Here's how the part is built. I have some questions about the finished solid (model axes, mm). Face numbers are marked on the shaded views. Round coordinates to 2 decimals unless told otherwise and drop trailing zeros. Loops run counter-clockwise (first coordinate to the right, second up) from the corner with the lowest first, then second, coordinate; pieces in that order, holes last. Notation, with made-up numbers: (18, 19.5) -> (36, 19.5) arc R26 ccw to (36, 40.5) -> close; hole circle Ø3 at (57, 55). An arc over 180 degrees is marked (long way). Use one line per item in the form item = value. Start each with the question number.
Item 1: If we section it at D-D (z = 0.25): Write out the boundary of the cut face in (x, y), then the cut area to 3 significant figures.
Item 2: If we section it at A-A (y = 8): Write out the boundary of the cut face in (x, z), then the cut area to 3 significant figures.
Item 3: If we section it at B-B (z = 4.75): Write out the boundary of the cut face in (x, y).
Item 4: If we section it at C-C (x = 27.5): Write out the boundary of the cut face in (y, z), then the cut area to 3 significant figures.
Item 5: I'm going to push flat-ended pins straight in: pin 1 Ø6 at (x, z) = (18.5, -3) entering from -Y; pin 2 Ø8 at (x, y) = (8, 8) entering from +Z. Where does each tip first touch, or does it pass through?
Item 6: Thinking about a two-plate mould opening in Y: for the marked faces 1, 2 and 3, which applies, released by +Y, released by -Y, zero draft, split by the parting line, or undercut?
Item 7: If I drill on L1, parallel to X at y = 36, z = -4.5; L2, parallel to X at y = 8, z = 2.75; L3, parallel to Y at x = 45, z = -5, over which ranges is the centre line in solid material (lowest first)? Write a range as [from, to].
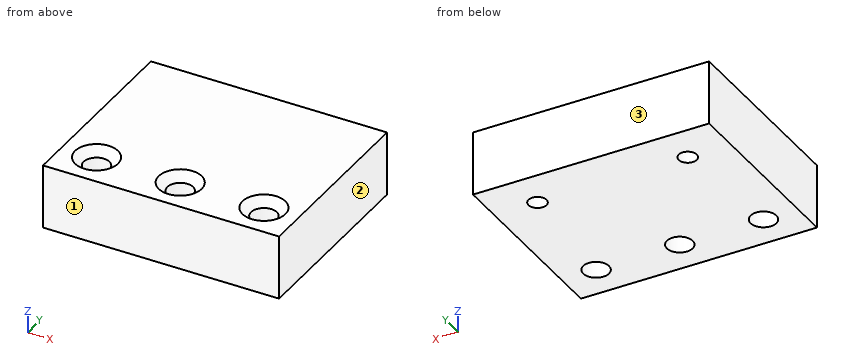
```python
from build123d import *

# Parameters (mm, degrees)
SKETCH1_W                       = 55
SKETCH1_H                       = 45
BOSS_EXTRUDE1_DEPTH             = 7.5
F_6_0MM_DOWEL_HOLE1_D           = 6
F_6_0MM_DOWEL_HOLE1_CSINK_D     = 10
F_6_0MM_DOWEL_HOLE1_CSINK_ANGLE = 90
TAP_DRILL_FOR_M5X0_8_TAP2_D     = 4.2
TAP_DRILL_FOR_M5X0_8_TAP2_DEPTH = 10
TAP_DRILL_FOR_M5X0_8_TAP2_TIP   = 1.2618073


with BuildPart() as part:
    # Sketch1 → Boss-Extrude1 (new body, symmetric)
    with BuildSketch(Plane.XY):
        with Locations((27.5, 22.5)):
            Rectangle(SKETCH1_W, SKETCH1_H)
    extrude(amount=BOSS_EXTRUDE1_DEPTH, both=True)

    # Ø6.0mm Dowel Hole1 (through all)
    with Locations(Plane(origin=(8, 8, 7.5), x_dir=(1, 0, 0), z_dir=(0, 0, 1))):
        with Locations((0, 0), (19.5, 0), (39, 0)):
            CounterSinkHole(F_6_0MM_DOWEL_HOLE1_D / 2, F_6_0MM_DOWEL_HOLE1_CSINK_D / 2, counter_sink_angle=F_6_0MM_DOWEL_HOLE1_CSINK_ANGLE)

    # Tap Drill for M5x0.8 Tap2
    with Locations(Plane(origin=(45, 36, -7.5), x_dir=(-1, 0, 0), z_dir=(0, 0, -1))):
        with Locations((0, 0), (35, 0)):
            Hole(TAP_DRILL_FOR_M5X0_8_TAP2_D / 2, depth=TAP_DRILL_FOR_M5X0_8_TAP2_DEPTH)
            with Locations((0, 0, -(TAP_DRILL_FOR_M5X0_8_TAP2_DEPTH + TAP_DRILL_FOR_M5X0_8_TAP2_TIP / 2))):  # 118° drill point
                Cone(0, TAP_DRILL_FOR_M5X0_8_TAP2_D / 2, TAP_DRILL_FOR_M5X0_8_TAP2_TIP, mode=Mode.SUBTRACT)


solid = part.part
```
Values found:
q1.outline = (0, 0) -> (55, 0) -> (55, 45) -> (0, 45) -> close; hole circle Ø6 at (8, 8); hole circle Ø4.2 at (10, 36); hole circle Ø6 at (27.5, 8); hole circle Ø4.2 at (45, 36); hole circle Ø6 at (47, 8)
q1.area = 2,360 mm2
q2.outline = (0, -7.5) -> (5, -7.5) -> (5, 5.5) -> (3, 7.5) -> (0, 7.5) -> close; (11, -7.5) -> (24.5, -7.5) -> (24.5, 5.5) -> (22.5, 7.5) -> (13, 7.5) -> (11, 5.5) -> close; (30.5, -7.5) -> (44, -7.5) -> (44, 5.5) -> (42, 7.5) -> (32.5, 7.5) -> (30.5, 5.5) -> close; (50, -7.5) -> (55, -7.5) -> (55, 7.5) -> (52, 7.5) -> (50, 5.5) -> close
q2.area = 543 mm2
q3.outline = (0, 0) -> (55, 0) -> (55, 45) -> (0, 45) -> close; hole circle Ø6 at (8, 8); hole circle Ø6 at (27.5, 8); hole circle Ø6 at (47, 8)
q4.outline = (0, -7.5) -> (5, -7.5) -> (5, 5.5) -> (3, 7.5) -> (0, 7.5) -> close; (11, -7.5) -> (45, -7.5) -> (45, 7.5) -> (13, 7.5) -> (11, 5.5) -> close
q4.area = 581 mm2
q5.pin_1 = 0
q5.pin_2 = 6.5
q6.face_1 = released by -Y
q6.face_2 = zero draft
q6.face_3 = released by +Y
q7.L1 = [0, 7.9], [12.1, 42.9], [47.1, 55]
q7.L2 = [0, 5], [11, 24.5], [30.5, 44], [50, 55]
q7.L3 = [0, 5.76], [10.24, 33.9], [38.1, 45]
